Source: CAD feature listing. Evaluate the final solid. Frame: model axes, mm. Give positions to 0.01 mm unless a question says otherwise; leave off trailing zeros. Write each loop counter-clockwise with the first axis right and the second up, starting at its lowest first coordinate (ties: lowest second). Pieces come first, ordered by that corner, then holes. Notation, with made-up numbers: M 39,61.25 L 70,61.25 A16 ccw 70,66.25 Z; hole C 71.5,2 d1. An arc over 180 degrees is marked long. Return JSON: item names as keys, results as strings.
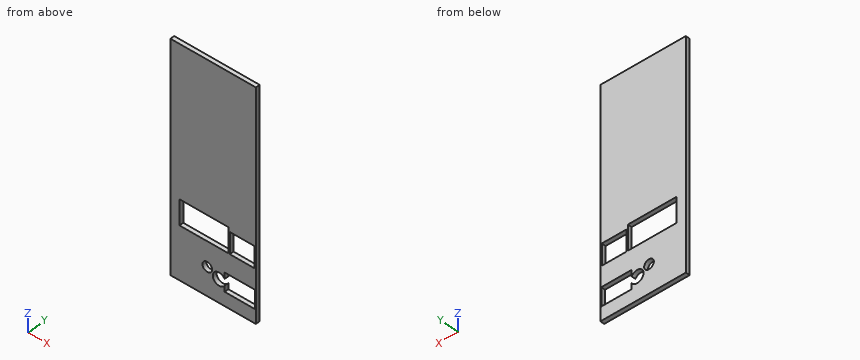
Autodesk Inventor part; units mm, degrees
ref_plane "YZ Plane" through (0, 0, 0) normal (1, 0, 0) x (0, 1, 0)
ref_plane "XZ Plane" through (0, 0, 0) normal (0, 1, 0) x (-1, 0, 0)
ref_plane "XY Plane" through (0, 0, 0) normal (0, 0, 1) x (1, 0, 0)
sketch "Sketch1" plane through (0, 0, 0) normal (0, 1, 0) x (-1, 0, 0)
  line L0 (0, 0) -> (62, 0)
  line L1 (62, 0) -> (62, -165)
  line L2 (62, -165) -> (0, -165)
  line L3 (0, -165) -> (0, 0)
  dimension "d0" = 165
  dimension "d1" = 62
extrude "Extrusion1" add sketch "Sketch1" along normal blind 3
sketch "Sketch2" plane through (0, 3, 0) normal (0, 1, 0) x (1, 0, 0)
  line L0 (-62, 165) -> (-62, 0)
  line L1 (3, 165) -> (-127, 165)
  circle A0 centre (-26.65, 148.375) radius 3.125
  line L2 (-18.9147, 111.2) -> (-1.0147, 111.2)
  line L3 (-1.0147, 111.2) -> (-1.0147, 126.7)
  line L4 (-1.0147, 126.7) -> (-18.9147, 126.7)
  line L5 (-18.9147, 126.7) -> (-18.9147, 111.2)
  line L6 (-17.6147, 112.2) -> (-2.3147, 112.2)
  line L7 (-7.804, 125.7) -> (-2.9647, 125.7)
  line L8 (-2.0147, 125.4) -> (-2.0147, 112.5)
  line L9 (-17.9147, 112.5) -> (-17.9147, 125.4)
  line L10 (-19.9657, 108.4) -> (-55.3657, 108.4)
  line L11 (-55.3657, 108.4) -> (-55.3657, 126.65)
  line L12 (-55.3657, 126.65) -> (-19.9657, 126.65)
  line L13 (-19.9657, 126.65) -> (-19.9657, 108.4)
  line L14 (-33.4157, 109.4) -> (-23.5157, 109.4)
  line L15 (-51.8157, 109.4) -> (-41.9157, 109.4)
  line L16 (-54.3657, 123.1) -> (-54.3657, 111.95)
  line L17 (-46.9157, 125.65) -> (-51.8157, 125.65)
  line L18 (-23.5157, 125.65) -> (-28.4157, 125.65)
  line L19 (-20.9657, 111.95) -> (-20.9657, 123.1)
  circle A1 centre (-26.65, 148.375) radius 4.625
  circle A2 centre (-35.25, 144.5) radius 3.5
  circle A3 centre (-35.25, 144.5) radius 2.5
  line L20 (-0.65, 141.5) -> (-22.65, 141.5)
  line L21 (-22.65, 141.5) -> (-22.65, 155)
  line L22 (-22.65, 155) -> (-0.65, 155)
  line L23 (-0.65, 155) -> (-0.65, 141.5)
  line L24 (-21.65, 142) -> (-1.65, 142)
  line L25 (-1.65, 142) -> (-1.65, 153)
  line L26 (-21.65, 153) -> (-1.65, 153)
  line L27 (-21.65, 142) -> (-21.65, 153)
  line L28 (0, 165) -> (-62, 165)
  line L29 (-62, 165) -> (-62, 0)
  point P0 (-35.25, 147)
  point P1 (-21.65, 147.5)
  point P2 (-22.65, 150.6968)
  point P3 (-22.65, 146.0532)
  dimension "d4" = 1
  dimension "d5" = 1
  dimension "d6" = 1
  dimension "d7" = 1
  dimension "d8" = 1
  dimension "d9" = 1
  dimension "d10" = 1
  dimension "d11" = 1
  dimension "d12" = 1.5
  dimension "d13" = 1
  dimension "d14" = 0.5
  dimension "d15" = 2
  dimension "d16" = 1
  dimension "d17" = 1
  dimension "d18" = 9.25
  dimension "d19" = 7
  dimension "d20" = 39.3
  dimension "d21" = 53.8
  dimension "d22" = 10
  dimension "d23" = 23.5
  dimension "d24" = 39.35
  dimension "d25" = 55.6
  dimension "d26" = 39.35
  dimension "d27" = 55.6
  dimension "d28" = 0.3647
  dimension "d29" = 17.2647
  dimension "d30" = 19.3157
  dimension "d31" = 21
  dimension "d32" = 53.7157
  dimension "d33" = 61.35
  dimension "d36" = 3.65
  dimension "d37" = 39.6
  dimension "d38" = 52.5
  dimension "d39" = 1.6647
  dimension "d40" = 2.3147
  dimension "d41" = 7.154
  dimension "d42" = 16.9647
  dimension "d43" = 39.6
  dimension "d44" = 52.5
  dimension "d45" = 41.9
  dimension "d46" = 53.05
  dimension "d47" = 22.8657
  dimension "d48" = 22.8657
  dimension "d49" = 26
  dimension "d50" = 27.7657
  dimension "d51" = 32.7657
  dimension "d52" = 18
  dimension "d53" = 34.6
  dimension "d54" = 34.6
  dimension "d55" = 41.2657
  dimension "d56" = 46.2657
  dimension "d57" = 51.1657
  dimension "d58" = 51.1657
  dimension "d59" = 41.9
  dimension "d60" = 53.05
  dimension "d61" = 0
  dimension "d62" = 165
  dimension "d63" = 126.35
extrude "Extrusion2" cut sketch "Sketch2" against normal through all contours A0 | L5 L4 L3 L2 | L10 L11 L12 L13 | A1 L21 | A1 L21 L22 L23 L20 | L21 A1 | A2 | A3 | L27 L26 L25 L24
properties part number "acrylicBackPanel"
1) Cut plane C-C, the plane x = -13. Return the cut outline in (y, z), then the cut area to 3 significant figures.
Numbers:
{"outline": "M 0,-165 L 3,-165 L 3,-155 L 0,-155 Z; M 0,-141.5 L 3,-141.5 L 3,-126.7 L 0,-126.7 Z; M 0,-111.2 L 3,-111.2 L 3,0 L 0,0 Z", "area": "408 mm²"}
2) Cut plane D-D, the plane x = -26.65. Return the cut outline in (y, z), then the cut area to 4 significant figures.
Numbers:
{"outline": "M 0,-165 L 3,-165 L 3,-153 L 0,-153 Z; M 0,-143.75 L 3,-143.75 L 3,-126.65 L 0,-126.65 Z; M 0,-108.4 L 3,-108.4 L 3,0 L 0,0 Z", "area": "412.5 mm²"}
3) Contact query for a flat-ended pin moving along its axis: pin 1 Ø5.5 at (x, z) = (-35.25, -144.5) entering from -Y. Output: stop coordinate, or through.
Numbers:
{"pin 1": "passes through"}
4) Cut plane A-A, the plane x = -46. Return the cut outline in (y, z).
Numbers:
{"outline": "M 0,-165 L 3,-165 L 3,-126.65 L 0,-126.65 Z; M 0,-108.4 L 3,-108.4 L 3,0 L 0,0 Z"}
5) Line query: line 1 (X direction, y = 2.2, z = -122); line 2 (Z direction, x = -26.65, y = 2.3); line 3 (Z direction, x = -35.25, y = 1.7). Output: solid intervals per line, ascending. Write a range as [from, to].
Numbers:
{"line 1": "x = [-62, -55.37], [-19.97, -18.91], [-1.01, 0]", "line 2": "z = [-165, -153], [-143.75, -126.65], [-108.4, 0]", "line 3": "z = [-165, -148], [-141, -126.65], [-108.4, 0]"}
6) Cut plane B-B, the plane y = 2.4. Return the cut outline in (x, z) (3 decimals), then the cut area to 3 significant figures.
Numbers:
{"outline": "M -62,-165 L 0,-165 L 0,0 L -62,0 Z; hole M -55.366,-126.65 L -19.966,-126.65 L -19.966,-108.4 L -55.366,-108.4 Z; hole C -35.25,-144.5 d7; hole M -22.65,-155 L -0.65,-155 L -0.65,-141.5 L -22.65,-141.5 L -22.65,-146.053 A4.625 ccw long -22.65,-150.697 Z; hole M -18.915,-126.7 L -1.015,-126.7 L -1.015,-111.2 L -18.915,-111.2 Z", "area": "8,910 mm²"}
